Source: CAD feature listing. Evaluate the final solid. Frame: model axes, mm. Round coordinates to 2 decimals unless told otherwise and drop trailing zeros. Loops run counter-clockwise (first coordinate to the right, second up) from the corner with the lowest first, then second, coordinate; pieces in that order, holes last. Notation, with made-up numbers: M 49,38 L 88,38 A21 cw 88,47 Z; hole C -14.5,50.5 d1. An arc over 180 degrees is marked long. Answer as a JSON object with one key per item and string values.
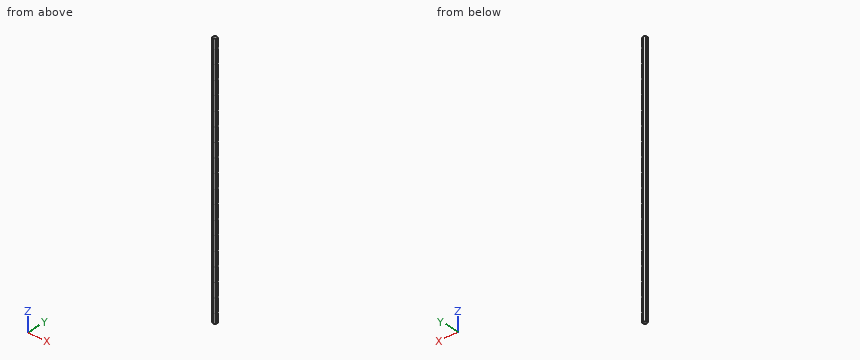
from build123d import *

# Parameters (mm, degrees)
BOSS_EXTRUDE1_DEPTH                             = 1100
CBORE_FOR_M5_SOCKET_HEAD_CAP_SCREW1_D           = 5.5
CBORE_FOR_M5_SOCKET_HEAD_CAP_SCREW1_CBORE_D     = 10
CBORE_FOR_M5_SOCKET_HEAD_CAP_SCREW1_CBORE_DEPTH = 5
LPATTERN1_COUNT                                 = 18
LPATTERN1_PITCH                                 = 60


with BuildPart() as part:
    # Sketch1 → Boss-Extrude1 (new body)
    with BuildSketch(Plane.XY):
        Polygon((0, -9.237604307), (8, -4.618802154), (8, 4.618802154), (0, 9.237604307), (-8, 4.618802154), (-8, -4.618802154), align=None)
    extrude(amount=BOSS_EXTRUDE1_DEPTH)

    # CBORE for M5 Socket Head Cap Screw1 (through all)
    with Locations(Plane(origin=(8, 0, 1060), x_dir=(0, 1, 0), z_dir=(1, 0, 0))):
        with Locations((0, 0)):
            cbore_for_m5_socket_head_cap_screw1 = CounterBoreHole(CBORE_FOR_M5_SOCKET_HEAD_CAP_SCREW1_D / 2, CBORE_FOR_M5_SOCKET_HEAD_CAP_SCREW1_CBORE_D / 2, CBORE_FOR_M5_SOCKET_HEAD_CAP_SCREW1_CBORE_DEPTH)

    # LPattern1: CBORE for M5 Socket Head Cap Screw1 ×18
    with Locations(*[(0, 0, -i * LPATTERN1_PITCH) for i in range(1, LPATTERN1_COUNT)]):
        add(cbore_for_m5_socket_head_cap_screw1, mode=Mode.SUBTRACT)


solid = part.part
Item 1: Line query: probe 1 along X at (y, z) = (-6.5, 74); probe 2 along Y at (x, z) = (-1.5, 1060); probe 3 along Y at (x, z) = (-4, 220). Output: solid intervals per line, ascending. Write a range as from..to.
Answer sheet:
{"probe 1": "x = -4.74..4.74", "probe 2": "y = -8.37..-2.75, 2.75..8.37", "probe 3": "y = -6.93..-2.75, 2.75..6.93"}
Item 2: Section B-B on x = -3.5. Give the number of separate pieces and of enclosed holes in the cut face, then the cut area to 3 significant figures.
Answer sheet:
{"separate pieces": "1", "enclosed holes": "18", "area": "15,400 mm²"}
Item 3: Section A-A on z = 903. Return the cut outline in (x, y), then the cut area to 3 significant figures.
Answer sheet:
{"outline": "M -8,-4.62 L 0,-9.24 L 8,-4.62 L 8,4.62 L 0,9.24 L -8,4.62 Z", "area": "222 mm²"}
Item 4: Contact query for flat-ended pins moving along their axis: pin 1 Ø6.5 at (y, z) = (0, 220) entering from +X; pin 2 Ø5 at (y, z) = (0, 700) entering from -X; pin 3 Ø11 at (y, z) = (2, 582) entering from +X; pin 4 Ø1 at (y, z) = (-7.5, 351) entering from -X. Output: stop coordinate, or through.
Answer sheet:
{"pin 1": "stops at x = 3", "pin 2": "passes through", "pin 3": "stops at x = 8", "pin 4": "stops at x = -3.88"}
